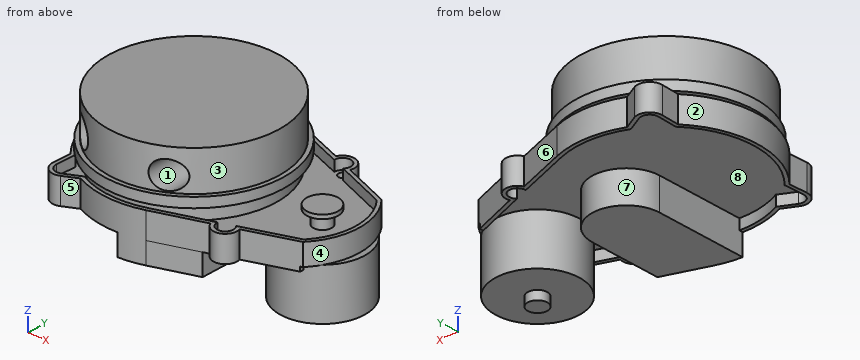
```python
from build123d import *

# Parameters (mm, degrees)
SKETCH_2_R               = 32.8
EXTRUDE_1_DEPTH          = 15.2
SKETCH_5_R               = 34.43969611
EXTRUDE_2_DEPTH          = 3.765573
SKETCH_7_R               = 31.937051091
EXTRUDE_3_DEPTH          = 0.8
SKETCH_8_R               = 31.627841621
EXTRUDE_4_DEPTH          = 4.8
EXTRUDE_6_DEPTH          = 2
EXTRUDE_START            = 4
EXTRUDE_7_DEPTH          = 4
EXTRUDE_8_DEPTH          = 6
CUT_EXTRUDE_1_DEPTH      = 1.7
SKETCH_14_R              = 3.5
EXTRUDE_9_DEPTH          = 5
SKETCH_15_R              = 6
EXTRUDE_10_DEPTH         = 1.5
EXTRUDE_START_2          = 2.3
SKETCH_16_R              = 3.5
EXTRUDE_11_DEPTH         = 2.3
SKETCH_17_R              = 16.25
EXTRUDE_12_DEPTH         = 19.5
SKETCH_18_R              = 3.75
EXTRUDE_13_DEPTH         = 3.43
EXTRUDE_14_DEPTH         = 12.23
CUT_EXTRUDE_2_DEPTH      = 81.031402587
CUT_EXTRUDE_2_DEPTH_BACK = 81.031402587
SKETCH_20_R              = 1.6
SKETCH_21_R              = 5.25
CUT_EXTRUDE_3_DEPTH      = 20


with BuildPart() as part:
    # 스케치2 → 보스-돌출1 (new body)
    with BuildSketch(Plane.XY):
        with Locations(Location((0, 0, 0), (0, 0, 180))):
            Circle(SKETCH_2_R)
    extrude(amount=EXTRUDE_1_DEPTH)

    # 스케치5 → 보스-돌출2 (add)
    with BuildSketch(Plane.XY):
        Circle(SKETCH_5_R)
    extrude(amount=-EXTRUDE_2_DEPTH)

    # 스케치7 → 보스-돌출3 (add)
    with BuildSketch(Plane(origin=(0, 0, -3.765572979), x_dir=(-1, 0, 0), z_dir=(0, 0, -1))):
        Circle(SKETCH_7_R)
    extrude(amount=EXTRUDE_3_DEPTH)

    # 스케치8 → 보스-돌출4 (add)
    with BuildSketch(Plane(origin=(0, 0, -4.565572979), x_dir=(-1, 0, 0), z_dir=(0, 0, -1))):
        Circle(SKETCH_8_R)
    extrude(amount=EXTRUDE_4_DEPTH)

    # 스케치10 → 보스-돌출6 (add)
    with BuildSketch(Plane(origin=(0, 0, -9.365572979), x_dir=(-1, 0, 0), z_dir=(0, 0, -1))):
        with BuildLine():
            Line((-30.830427643, -26.692532528), (-11.928490857, -33.435925378))
            ThreePointArc((-11.928490857, -33.435925378), (1.386891377, -35.472898561), (14.502591336, -32.402543797))
            Line((14.502591336, -32.402543797), (19.833940849, -35.171113491))
            ThreePointArc((19.833940849, -35.171113491), (24.525943879, -34.963534725), (26.69566429, -30.798166229))
            Line((26.69566429, -30.798166229), (26.392377939, -23.742206863))
            ThreePointArc((26.392377939, -23.742206863), (35.5, 0), (26.392377939, 23.742206863))
            Line((26.392377939, 23.742206863), (26.69566429, 30.798166229))
            ThreePointArc((26.69566429, 30.798166229), (24.525943879, 34.963534725), (19.833940849, 35.171113491))
            Line((19.833940849, 35.171113491), (14.502591336, 32.402543797))
            ThreePointArc((14.502591336, 32.402543797), (1.386891377, 35.472898561), (-11.928490857, 33.435925378))
            Line((-11.928490857, 33.435925378), (-30.830427643, 26.692532528))
            ThreePointArc((-30.830427643, 26.692532528), (-36.575929002, 29.215026427), (-39.257220366, 23.541893434))
            Line((-39.257220366, 23.541893434), (-57.703429714, 16.761281639))
            ThreePointArc((-57.703429714, 16.761281639), (-64.057876626, 0), (-57.703429714, -16.761281639))
            Line((-57.703429714, -16.761281639), (-39.257220366, -23.541893434))
            ThreePointArc((-39.257220366, -23.541893434), (-36.575929002, -29.215026427), (-30.830427643, -26.692532528))
        make_face()
    extrude(amount=EXTRUDE_6_DEPTH)

    # 스케치12 → 보스-돌출7 (add)
    with BuildSketch(Plane.XY.offset(-9.365572979).offset(EXTRUDE_START)):
        with BuildLine():
            Line((-26.392377939, -23.742206863), (-26.69566429, -30.798166229))
            ThreePointArc((-26.69566429, -30.798166229), (-24.525943879, -34.963534725), (-19.833940849, -35.171113491))
            Line((-19.833940849, -35.171113491), (-14.502591336, -32.402543797))
            ThreePointArc((-14.502591336, -32.402543797), (-1.386891377, -35.472898561), (11.928490857, -33.435925378))
            Line((11.928490857, -33.435925378), (30.830427643, -26.692532528))
            ThreePointArc((30.830427643, -26.692532528), (36.575929002, -29.215026427), (39.257220366, -23.541893434))
            Line((39.257220366, -23.541893434), (57.703429714, -16.761281639))
            ThreePointArc((57.703429714, -16.761281639), (64.057876626, 0), (57.703429714, 16.761281639))
            Line((57.703429714, 16.761281639), (39.257220366, 23.541893434))
            ThreePointArc((39.257220366, 23.541893434), (36.575929002, 29.215026427), (30.830427643, 26.692532528))
            Line((30.830427643, 26.692532528), (11.928490857, 33.435925378))
            ThreePointArc((11.928490857, 33.435925378), (-1.386891377, 35.472898561), (-14.502591336, 32.402543797))
            Line((-14.502591336, 32.402543797), (-19.833940849, 35.171113491))
            ThreePointArc((-19.833940849, 35.171113491), (-24.525943879, 34.963534725), (-26.69566429, 30.798166229))
            Line((-26.69566429, 30.798166229), (-26.392377939, 23.742206863))
            ThreePointArc((-26.392377939, 23.742206863), (-35.5, 0), (-26.392377939, -23.742206863))
        make_face()
        with BuildLine():
            Line((-24.968823812, -23.224294122), (-25.296955778, -30.858286926))
            ThreePointArc((-25.296955778, -30.858286926), (-23.773535064, -33.78290736), (-20.479149958, -33.928654153))
            Line((-20.479149958, -33.928654153), (-14.540295767, -30.844607292))
            ThreePointArc((-14.540295767, -30.844607292), (-1.667327059, -34.059213445), (11.458071499, -32.117325504))
            Line((11.458071499, -32.117325504), (31.905073194, -24.822720374))
            ThreePointArc((31.905073194, -24.822720374), (36.103194509, -27.897060903), (37.193109232, -22.809047719))
            Line((37.193109232, -22.809047719), (56.884193028, -15.570834571))
            ThreePointArc((56.884193028, -15.570834571), (62.657876626, 0), (56.884193028, 15.570834571))
            Line((56.884193028, 15.570834571), (37.193109232, 22.809047719))
            ThreePointArc((37.193109232, 22.809047719), (36.103194509, 27.897060903), (31.905073194, 24.822720374))
            Line((31.905073194, 24.822720374), (11.458071499, 32.117325504))
            ThreePointArc((11.458071499, 32.117325504), (-1.667327059, 34.059213445), (-14.540295767, 30.844607292))
            Line((-14.540295767, 30.844607292), (-20.479149958, 33.928654153))
            ThreePointArc((-20.479149958, 33.928654153), (-23.773535064, 33.78290736), (-25.296955778, 30.858286926))
            Line((-25.296955778, 30.858286926), (-24.968823812, 23.224294122))
            ThreePointArc((-24.968823812, 23.224294122), (-34.1, 0), (-24.968823812, -23.224294122))
        make_face(mode=Mode.SUBTRACT)
    extrude(amount=-EXTRUDE_7_DEPTH)

    # 스케치12<2> → 보스-돌출8 (add)
    with BuildSketch(Plane.XY.offset(-9.365572979)):
        with BuildLine():
            Line((-26.392377939, -23.742206863), (-26.69566429, -30.798166229))
            ThreePointArc((-26.69566429, -30.798166229), (-24.525943879, -34.963534725), (-19.833940849, -35.171113491))
            Line((-19.833940849, -35.171113491), (-14.502591336, -32.402543797))
            ThreePointArc((-14.502591336, -32.402543797), (-1.386891377, -35.472898561), (11.928490857, -33.435925378))
            Line((11.928490857, -33.435925378), (30.830427643, -26.692532528))
            ThreePointArc((30.830427643, -26.692532528), (36.575929002, -29.215026427), (39.257220366, -23.541893434))
            Line((39.257220366, -23.541893434), (57.703429714, -16.761281639))
            ThreePointArc((57.703429714, -16.761281639), (64.057876626, 0), (57.703429714, 16.761281639))
            Line((57.703429714, 16.761281639), (39.257220366, 23.541893434))
            ThreePointArc((39.257220366, 23.541893434), (36.575929002, 29.215026427), (30.830427643, 26.692532528))
            Line((30.830427643, 26.692532528), (11.928490857, 33.435925378))
            ThreePointArc((11.928490857, 33.435925378), (-1.386891377, 35.472898561), (-14.502591336, 32.402543797))
            Line((-14.502591336, 32.402543797), (-19.833940849, 35.171113491))
            ThreePointArc((-19.833940849, 35.171113491), (-24.525943879, 34.963534725), (-26.69566429, 30.798166229))
            Line((-26.69566429, 30.798166229), (-26.392377939, 23.742206863))
            ThreePointArc((-26.392377939, 23.742206863), (-35.5, 0), (-26.392377939, -23.742206863))
        make_face()
        with BuildLine():
            Line((-24.968823812, -23.224294122), (-25.296955778, -30.858286926))
            ThreePointArc((-25.296955778, -30.858286926), (-23.773535064, -33.78290736), (-20.479149958, -33.928654153))
            Line((-20.479149958, -33.928654153), (-14.540295767, -30.844607292))
            ThreePointArc((-14.540295767, -30.844607292), (-1.667327059, -34.059213445), (11.458071499, -32.117325504))
            Line((11.458071499, -32.117325504), (31.905073194, -24.822720374))
            ThreePointArc((31.905073194, -24.822720374), (36.103194509, -27.897060903), (37.193109232, -22.809047719))
            Line((37.193109232, -22.809047719), (56.884193028, -15.570834571))
            ThreePointArc((56.884193028, -15.570834571), (62.657876626, 0), (56.884193028, 15.570834571))
            Line((56.884193028, 15.570834571), (37.193109232, 22.809047719))
            ThreePointArc((37.193109232, 22.809047719), (36.103194509, 27.897060903), (31.905073194, 24.822720374))
            Line((31.905073194, 24.822720374), (11.458071499, 32.117325504))
            ThreePointArc((11.458071499, 32.117325504), (-1.667327059, 34.059213445), (-14.540295767, 30.844607292))
            Line((-14.540295767, 30.844607292), (-20.479149958, 33.928654153))
            ThreePointArc((-20.479149958, 33.928654153), (-23.773535064, 33.78290736), (-25.296955778, 30.858286926))
            Line((-25.296955778, 30.858286926), (-24.968823812, 23.224294122))
            ThreePointArc((-24.968823812, 23.224294122), (-34.1, 0), (-24.968823812, -23.224294122))
        make_face(mode=Mode.SUBTRACT)
    extrude(amount=-EXTRUDE_8_DEPTH)

    # 스케치13 → 컷-돌출1 (cut)
    with BuildSketch(Plane(origin=(0, 0, -15.365572979), x_dir=(-1, 0, 0), z_dir=(0, 0, -1))):
        Polygon((-56.884193028, -15.570834571), (-56.884193028, 17.062423507), (-56.884193028, 21.549560303), (-68.095644454, 21.549560303), (-68.095644454, -21.067118875), (-56.884193028, -21.067118875), align=None)
    extrude(amount=-CUT_EXTRUDE_1_DEPTH, mode=Mode.SUBTRACT)

    # 스케치14 → 보스-돌출9 (add)
    with BuildSketch(Plane.XY.offset(-9.365572979)):
        with Locations(Location((50, 0, 0), (0, 0, 180))):
            Circle(SKETCH_14_R)
    extrude(amount=EXTRUDE_9_DEPTH)

    # 스케치15 → 보스-돌출10 (add)
    with BuildSketch(Plane.XY.offset(-4.365572979)):
        with Locations((50, 0)):
            Circle(SKETCH_15_R)
    extrude(amount=EXTRUDE_10_DEPTH)

    # 스케치16 → 보스-돌출11 (add)
    with BuildSketch(Plane(origin=(0, 0, -11.365572979), x_dir=(-1, 0, 0), z_dir=(0, 0, -1)).offset(EXTRUDE_START_2)):
        with Locations((-50, 0)):
            Circle(SKETCH_16_R)
    extrude(amount=-EXTRUDE_11_DEPTH)

    # 스케치17 → 보스-돌출12 (add)
    with BuildSketch(Plane(origin=(0, 0, -13.665572979), x_dir=(-1, 0, 0), z_dir=(0, 0, -1))):
        with Locations(Location((-50, 0, 0), (0, 0, 133.077401672))):
            Circle(SKETCH_17_R)
    extrude(amount=EXTRUDE_12_DEPTH)

    # 스케치18 → 보스-돌출13 (add)
    with BuildSketch(Plane(origin=(0, 0, -33.165572979), x_dir=(-1, 0, 0), z_dir=(0, 0, -1))):
        with Locations(Location((-50, 0, 0), (0, 0, 180))):
            Circle(SKETCH_18_R)
    extrude(amount=EXTRUDE_13_DEPTH)

    # 스케치19 → 보스-돌출14 (add)
    with BuildSketch(Plane(origin=(0, 0, -11.365572979), x_dir=(-1, 0, 0), z_dir=(0, 0, -1))):
        with BuildLine():
            Line((-28.5, 0), (-28.5, -27.523928235))
            Line((-28.5, -27.523928235), (-11.928490857, -33.435925378))
            ThreePointArc((-11.928490857, -33.435925378), (-7.281580797, -34.745195079), (-2.5, -35.411862419))
            Line((-2.5, -35.411862419), (-2.5, 0))
            ThreePointArc((-2.5, 0), (-15.5, 13), (-28.5, 0))
        make_face()
    extrude(amount=EXTRUDE_14_DEPTH)

    # 스케치20 → 컷-돌출2 (cut, two sides: drawn at the far end of the back side and taken through both)
    with BuildSketch(Plane.XY.offset(-9.365572979).offset(-CUT_EXTRUDE_2_DEPTH_BACK)):
        with Locations(Location((35, -25, 0), (0, 0, 180))):
            Circle(SKETCH_20_R)
        with Locations(Location((-22, -31, 0), (0, 0, 180))):
            Circle(SKETCH_20_R)
        with Locations(Location((35, 25, 0), (0, 0, 180))):
            Circle(SKETCH_20_R)
        with Locations(Location((-22, 31, 0), (0, 0, 180))):
            Circle(SKETCH_20_R)
    extrude(amount=CUT_EXTRUDE_2_DEPTH + CUT_EXTRUDE_2_DEPTH_BACK, mode=Mode.SUBTRACT)

    # 스케치21 → 컷-돌출3 (cut)
    with BuildSketch(Plane(origin=(0, -33, 0), x_dir=(1, 0, 0), z_dir=(0, 1, 0))):
        with Locations(Location((15.9, -5.8, 0), (0, 0, 90))):
            Circle(SKETCH_21_R)
        with Locations(Location((-19.5, -5.8, 0), (0, 0, 90))):
            Circle(SKETCH_21_R)
    extrude(amount=CUT_EXTRUDE_3_DEPTH, mode=Mode.SUBTRACT)


solid = part.part
```
For this review, take the finished solid that the model builds, in its own axes (mm). Face numbers are marked on the shaded views. A direction names the side the tool comes from. Coordinates: 2 decimals unless noted, no trailing zeros. Write each loop counter-clockwise with the first axis right and the second up, starting at its lowest first coordinate (ties: lowest second). Pieces come first, ordered by that corner, then holes.
(1) Add section A-A on z = -21. Give the boundary of the cut face in (x, y).
(2) Tool access review of the marked faces 4, 5, 6, 7 and 8: name each direction out of +Z, -Z, +X, -X, +Y, -Y from which nothing blocks a thin tool from reaching the whole face with its end or side.
(3) Wall thickness on probe 1 along Y at (x, z) = (-22, -10); probe 2 along Y at (x, z) = (35, -10.8); probe 3 along Y at (x, z) = (35, -13): over which ranges is each line inside the solid? List them lowest first.
(4) The part is to be moulded in two halves that separate along X. For the marked faces 1, 2 and 3, say which applies: +X half, -X half, draft (parallel to the pull), parting line (faces both ways), or undercut.
(5) For pin 1 Ø6 at (x, y) = (-8, 15) entering from -Z; pin 2 Ø1 at (y, z) = (3, -12.5) entering from -X; pin 3 Ø6 at (y, z) = (-11.5, -18.5) entering from +X, all flat-tipped, find the tip position at first contact; note any pin that passes through.
(6) Add section B-B on x = 41. Give the boundary of the cut face in (y, z), then the cut area to 3 significant figures.
(7) Add section D-D on x = -6.5. Give the boundary of the cut face in (y, z).
Answer sheet:
1. outline: (2.5, -35.41) arc R35.5 ccw to (11.93, -33.44) - (28.5, -27.52) - (28.5, 0) arc R13 ccw to (2.5, 0) - close; circle Ø32.5 at (50, 0)
2. face 4: +Z, +X
2. face 5: +Z, -Z, -Y
2. face 6: +Z, -Z, +Y
2. face 7: -Z
2. face 8: none
3. probe 1: y = -35.7 to -32.6, -29.4 to 29.4, 32.6 to 35.7
3. probe 2: y = -29.5 to -26.6, -23.4 to 23.4, 26.6 to 29.5
3. probe 3: y = -29.5 to -28.1, 28.1 to 29.5
4. face 1: undercut
4. face 2: -X half
4. face 3: parting line
5. pin 1: stops at z = -11.37
5. pin 2: stops at x = -35.41
5. pin 3: stops at x = 63.85
6. outline: (-22.9, -15.37) - (-21.41, -15.37) - (-21.41, -11.37) - (21.41, -11.37) - (21.41, -15.37) - (22.9, -15.37) - (22.9, -5.37) - (21.41, -5.37) - (21.41, -9.37) - (-21.41, -9.37) - (-21.41, -5.37) - (-22.9, -5.37) - close; (-13.53, -33.17) - (13.53, -33.17) - (13.53, -13.67) - (-13.53, -13.67) - close
6. area: 643 mm2
7. outline: (-34.9, -15.37) - (-33.47, -15.37) - (-33.47, -11.37) - (33.47, -11.37) - (33.47, -15.37) - (34.9, -15.37) - (34.9, -5.37) - (33.47, -5.37) - (33.47, -9.37) - (30.95, -9.37) - (30.95, -4.57) - (31.27, -4.57) - (31.27, -3.77) - (33.82, -3.77) - (33.82, 0) - (32.15, 0) - (32.15, 15.2) - (-32.15, 15.2) - (-32.15, 0) - (-33.82, 0) - (-33.82, -3.77) - (-31.27, -3.77) - (-31.27, -4.57) - (-30.95, -4.57) - (-30.95, -9.37) - (-33.47, -9.37) - (-33.47, -5.37) - (-34.9, -5.37) - close
